Geometry check sheet. Reference: the model listing, model coordinates, mm. Face numbers are marked on the shaded views. A direction names the side the tool comes from. Round coordinates to 2 decimals unless told otherwise and drop trailing zeros. Write each loop counter-clockwise with the first axis right and the second up, starting at its lowest first coordinate (ties: lowest second). Pieces come first, ordered by that corner, then holes. Notation, with made-up numbers: (44.25, -1.75) - (103.25, -1.75) arc R36 ccw to (103.25, 33.25) - close; hole circle Ø1 at (-24.5, 5.5). An arc over 180 degrees is marked (long way). Return JSON: item names as keys, results as strings. Group by question number.
from build123d import *

# Parameters (mm, degrees)
F1_DEPTH = 25.4
F2_DEPTH = 50.8


with BuildPart() as f1:
    # F0 (on Top) → F1 (new body)
    with BuildSketch(Plane.XY):
        Polygon((88.838113, 51.116822), (38.042081, 26.351779), (38.042081, 0.951779), (88.838113, -23.813265), align=None)
    extrude(amount=F1_DEPTH)

    # F0 (on Top) → F2 (join)
    with BuildSketch(Plane.XY):
        Polygon((38.042081, 51.751779), (-63.557919, 51.751779), (-63.557919, -24.448221), (38.042081, -24.448221), (38.042081, 0.951779), (38.042081, 26.351779), align=None)
    extrude(amount=F2_DEPTH)


solid = f1.part
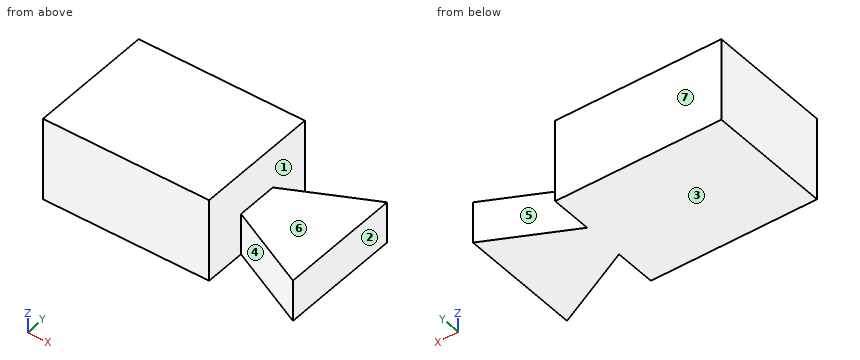
1. Depth check by flat-ended pin: pin 1 Ø4 at (x, y) = (-35, -6.5) entering from -Z; pin 2 Ø2 at (y, z) = (11, 44.5) entering from +X. Enter the tip coordinate at first touch or a pass-through.
2. Section check B-B (y = 41.5). Enter the section's corners in (x, z), and give its area (3 significant figures).
3. Section check A-A (z = 14.5). Enter the section's corners in (x, y).
4. Section check D-D (y = -13). Enter the section's corners in (x, z).
5. Material ranges on line 1 along Z through (x, y) = (70, -13.5); line 2 along X through (y, z) = (-2, 45.5); line 3 along X through (y, z) = (-15, 7), recorded low to high.
6. Section check C-C (y = 20). Enter the section's corners in (x, z).
7. Mould release check, pull along X, two halves, no side actions. Record for the marked faces 1, 2 and 3: pulls with the +X half, pulls with the -X half, needs draft (parallel to the pull), parting line crosses it, or undercut.
8. Tool access check on the marked faces 4, 5, 6 and 7. Record the directions out of +Z, -Z, +X, -X, +Y, -Y that give a thin tool (end or side, any length) a straight path to the whole face; none if there is none.
Result sheet:
{
 "1": {"pin 1": "stops at z = 0", "pin 2": "stops at x = 38.04"},
 "2": {"outline": "(-63.56, 0) - (38.04, 0) - (38.04, 50.8) - (-63.56, 50.8) - close; (69.11, 0) - (88.84, 0) - (88.84, 25.4) - (69.11, 25.4) - close", "area": "5,660 mm²"},
 "3": {"outline": "(-63.56, -24.45) - (38.04, -24.45) - (38.04, 0.95) - (88.84, -23.81) - (88.84, 51.12) - (38.04, 26.35) - (38.04, 51.75) - (-63.56, 51.75) - close"},
 "4": {"outline": "(-63.56, 0) - (38.04, 0) - (38.04, 50.8) - (-63.56, 50.8) - close; (66.66, 0) - (88.84, 0) - (88.84, 25.4) - (66.66, 25.4) - close"},
 "5": {"line 1": "z = 0 to 25.4", "line 2": "x = -63.56 to 38.04", "line 3": "x = -63.56 to 38.04, 70.76 to 88.84"},
 "6": {"outline": "(-63.56, 0) - (88.84, 0) - (88.84, 25.4) - (38.04, 25.4) - (38.04, 50.8) - (-63.56, 50.8) - close"},
 "7": {"face 1": "undercut", "face 2": "pulls with the +X half", "face 3": "needs draft"},
 "8": {"face 4": "+Z, -Z, -Y", "face 5": "+Z, -Z, +Y", "face 6": "+Z, +X, +Y, -Y", "face 7": "+Z, -Z, +X, -X, +Y"}
}
